from build123d import *

# Parameters (mm, degrees)
F0_W      = 33.25091
F0_H      = 82.434542
F3_DEPTH  = 25.4
F1_R      = 16.625455
F4_DEPTH  = 25.4
F2_R      = 16.394546
F5_DEPTH  = 25.4
F6_R      = 6.38663
F6_R_2    = 6.732099
F7_DEPTH  = 25.401
F8_W      = 20.32
F8_H      = 52.416362
F9_DEPTH  = 50.8
F11_DEPTH = 26.786455
F12_W     = 10.16
F12_H     = 6.445338
F14_W     = 10.16
F14_H     = 6.445338
F16_R     = 3.356131
F17_DEPTH = 84.051907


with BuildPart() as f3:
    # F0 (on Top) → F3 (new body)
    with BuildSketch(Plane.XY):
        Rectangle(F0_W, F0_H)
    extrude(amount=F3_DEPTH)

    # F1 (on Top) → F4 (join)
    with BuildSketch(Plane.XY):
        with Locations((0, 41.217271)):
            Circle(F1_R)
    extrude(amount=F4_DEPTH)

    # F2 (on Top) → F5 (join)
    with BuildSketch(Plane.XY):
        with Locations((0, -41.217271)):
            Circle(F2_R)
    extrude(amount=F5_DEPTH)

    # F6 (on face) → F7 (cut, through all)
    with BuildSketch(Plane.XY.offset(25.4)):
        with Locations((0, 41.217271)):
            Circle(F6_R)
        with Locations((0, -41.217271)):
            Circle(F6_R_2)
    extrude(amount=-F7_DEPTH, mode=Mode.SUBTRACT)

    # F8 (on Top) → F9 (join)
    with BuildSketch(Plane.XY):
        Rectangle(F8_W, F8_H)
    extrude(amount=F9_DEPTH)

    # F10 (on face) → F11 (cut, through all)
    with BuildSketch(Plane.YZ.offset(10.16)):
        with BuildLine():
            Line((-19.762843, 50.8), (19.762843, 50.8))
            ThreePointArc((19.762843, 50.8), (0, 70.562843), (-19.762843, 50.8))
        make_face()
        with BuildLine():
            ThreePointArc((-19.762843, 50.8), (0, 31.037157), (19.762843, 50.8))
            Line((19.762843, 50.8), (-19.762843, 50.8))
        make_face()
    extrude(amount=-F11_DEPTH, mode=Mode.SUBTRACT)

    # F12 (on face) → F13 (revolve)
    with BuildSketch(Plane.XY.offset(50.8)):
        with Locations((5.08, 22.985512)):
            Rectangle(F12_W, F12_H)
    revolve(axis=Axis((0, 22.985512, 50.8), (0, -1, 0)))

    # F14 (on face) → F15 (revolve)
    with BuildSketch(Plane.XY.offset(50.8)):
        with Locations((-5.08, -22.985512)):
            Rectangle(F14_W, F14_H)
    revolve(axis=Axis((0, -22.985512, 50.8), (0, 1, 0)))

    # F16 (on face) → F17 (cut, through all)
    with BuildSketch(Plane.XZ.offset(26.208181)):
        with Locations((0, 50.8)):
            Circle(F16_R)
    extrude(amount=-F17_DEPTH, mode=Mode.SUBTRACT)


solid = f3.part
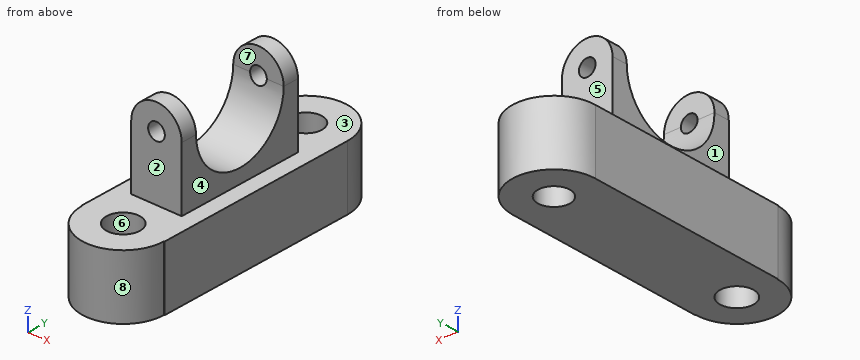
Input: part model. Units: mm. Frame: model coordinates. Face numbers are marked on the shaded views. A direction names the side the tool comes from. Give positions to 0.01 mm unless a question says otherwise; leave off trailing zeros. Write each loop counter-clockwise with the first axis right and the second up, starting at its lowest first coordinate (ties: lowest second). Pieces come first, ordered by that corner, then holes. Notation, with made-up numbers: M 25,7.25 L 64,7.25 A8 cw 64,11.25 Z; hole C 20,-28.5 d9. An arc over 180 degrees is marked long. Write item = value, one per line. Start each with the question number.
1) Cut plane C-C on z = 44.5. Return the cut outline in (x, y), then the cut area to 3 significant figures.
2) Cut plane A-A on x = 0. Return the cut outline in (y, z).
3) Cut plane B-B on y = 0. Return the cut outline in (x, z), then the cut area to 3 significant figures.
4) Draft query along X for the marked faces 6, 7 and 8. Return one class per face: +X half, -X half, draft (parallel to the pull), parting line (faces both ways), or undercut.
5) Cut plane D-D on z = 26.5. Return the cut outline in (x, y), then the cut area to 3 significant figures.
6) Material intervals for line 1 along Y through (x, z) = (0, 10.25); line 2 along Z through (x, y) = (0, 23); line 3 along Y through (x, z) = (-3.5, 13), sorted ascending. Write a range as [from, to].
7) Reachability of the marked faces 1, 2, 3, 4 and 5 from +Z, -Z, +X, -X, +Y, -Y: full face, straight path, thin tool, end or side. Return the list, or none.
8) First-contact query: pin 1 Ø6 at (x, z) = (-4.5, 41.5) entering from -Y; pin 2 Ø10 at (x, z) = (-11.5, 12) entering from +Y; pin 3 Ø8 at (x, z) = (0, 55) entering from +Y; pin 4 Ø7.5 at (x, y) = (0, 41.22) entering from -Z. Flat tips, straight axial feed; report the tip coordinate or a pass-through.
Solved:
q1.outline = M -10.16,-26.21 L 10.16,-26.21 L 10.16,-18.73 L -10.16,-18.73 Z; M -10.16,18.73 L 10.16,18.73 L 10.16,26.21 L -10.16,26.21 Z
q1.area = 304 mm2
q2.outline = M -57.61,0 L -47.95,0 L -47.95,25.4 L -57.61,25.4 Z; M -34.49,0 L 34.83,0 L 34.83,25.4 L 26.21,25.4 L 26.21,47.44 L 19.48,47.44 A19.76 cw -19.48,47.44 L -26.21,47.44 L -26.21,25.4 L -34.49,25.4 Z; M -26.21,54.16 L -19.76,54.16 L -19.76,60.96 L -26.21,60.96 Z; M 19.76,54.16 L 26.21,54.16 L 26.21,60.96 L 19.76,60.96 Z; M 47.6,0 L 57.84,0 L 57.84,25.4 L 47.6,25.4 Z
q3.outline = M -16.63,0 L 16.63,0 L 16.63,25.4 L 10.16,25.4 L 10.16,31.04 L -10.16,31.04 L -10.16,25.4 L -16.63,25.4 Z
q3.area = 959 mm2
q4.face_6 = undercut
q4.face_7 = draft
q4.face_8 = parting line
q5.outline = M -10.16,-26.21 L 10.16,-26.21 L 10.16,26.21 L -10.16,26.21 Z
q5.area = 1,070 mm2
q6.line_1 = [-57.61, -47.95], [-34.49, 34.83], [47.6, 57.84]
q6.line_2 = [0, 47.44], [54.16, 60.96]
q6.line_3 = [-57.23, -46.97], [-35.47, 35.88], [46.56, 57.47]
q7.face_1 = +Z, -X, +Y, -Y
q7.face_2 = +Z, +X, -X, -Y
q7.face_3 = +Z
q7.face_4 = +Z, +X, +Y, -Y
q7.face_5 = +Z, +X, -X, +Y
q8.pin_1 = -26.21
q8.pin_2 = 56.52
q8.pin_3 = 26.21
q8.pin_4 = through
